from build123d import *

# Parameters (mm, degrees)
F0_W     = 35
F0_H     = 35
F1_DEPTH = 3.5
F2_R     = 2
F3_DEPTH = 7.001
F4_R     = 5
F5_R     = 3.15
F6_DEPTH = 6.3
F7_R     = 2.5
F8_DEPTH = 13.301
F9_SIZE  = 1.4
F10_R    = 0.5


with BuildPart() as f1:
    # F0 (on Top) → F1 (new body, symmetric)
    with BuildSketch(Plane.XY):
        Rectangle(F0_W, F0_H)
    extrude(amount=F1_DEPTH, both=True)

    # F2 (on face) → F3 (cut, through all)
    with BuildSketch(Plane.XY.offset(3.5)):
        with Locations((-12.5, -12.9)):
            Circle(F2_R)
        with Locations((-12.5, 12.5)):
            Circle(F2_R)
        with Locations((12.5, 12.5)):
            Circle(F2_R)
        with Locations((12.5, -12.9)):
            Circle(F2_R)
    extrude(amount=-F3_DEPTH, mode=Mode.SUBTRACT)

    # F4
    f4_edges = [f1.edges().sort_by_distance(p)[0] for p in [
        (-17.5, 17.5, 0),
        (17.5, 17.5, 0),
        (17.5, -17.5, 0),
        (-17.5, -17.5, 0),
    ]]
    fillet(f4_edges, radius=F4_R)

    # F5 (on face) → F6 (join)
    with BuildSketch(Plane.XY.offset(3.5)):
        Circle(F5_R)
    extrude(amount=F6_DEPTH)

    # F7 (on face) → F8 (cut, through all)
    with BuildSketch(Plane.XY.offset(9.8)):
        Circle(F7_R)
    extrude(amount=-F8_DEPTH, mode=Mode.SUBTRACT)

    # F9
    f9_edges = [f1.edges().sort_by_distance(p)[0] for p in [
        (-14.5, -12.9, -3.5),
        (10.5, -12.9, -3.5),
        (10.5, 12.5, -3.5),
        (-14.5, 12.5, -3.5),
    ]]
    chamfer(f9_edges, length=F9_SIZE)

    # F10
    f10_edges = [f1.edges().sort_by_distance(p)[0] for p in [
        (-15.9, -12.9, -3.5),
        (-17.5, 0, -3.5),
    ]]
    fillet(f10_edges, radius=F10_R)


solid = f1.part
Design review of the part built by this model. Coordinates are the model's own, in mm. Coordinates: 2 decimals unless noted, no trailing zeros. Write each loop counter-clockwise with the first axis right and the second up, starting at its lowest first coordinate (ties: lowest second). Pieces come first, ordered by that corner, then holes. Notation, with made-up numbers: (10.25, -32.5) - (43.25, -32.5) arc R25 cw to (43.25, -13.5) - close; hole circle Ø7 at (-16.75, 69). An arc over 180 degrees is marked (long way). One line per item, written item: value.
1) Mouldability with a two-part tool opening along Y and no side actions: class faces 1 (the face through (-16.07, 16, 0.2)), 2 (the face through (-12.76, -10.917, 0.739)), 3 (the face through (0, 4, -3.5)) as +Y half, -Y half, draft (parallel to the pull), parting line (faces both ways), or undercut.
Answer sheet:
face 1: +Y half
face 2: undercut
face 3: draft
2) To check wall thickness, follow probe 1 along Y at (x, z) = (-12.5, 2.3); probe 2 along Z at (x, y) = (14, 4); probe 3 along Y at (x, z) = (-11, -2.25). State the ranges of each line that lie inside material, in increasing order.
Answer sheet:
probe 1: y = -17.5 to -14.9, -10.9 to 10.5, 14.5 to 17.5
probe 2: z = -3.5 to 3.5
probe 3: y = -17.5 to -14.44, -11.36 to 10.96, 14.04 to 17.5
3) Add section D-D (z = 8.25). State the section outline as (x, y) points.
Answer sheet:
outline: circle Ø6.3 at (0, 0); hole circle Ø5 at (0, 0)
4) Add section C-C (y = -0.5). State the section outline as (x, z) points, plus the area to 3 significant figures.
Answer sheet:
outline: (-17.5, -3) arc R0.5 ccw to (-17, -3.5) - (-2.45, -3.5) - (-2.45, 9.8) - (-3.11, 9.8) - (-3.11, 3.5) - (-17.5, 3.5) - close; (2.45, -3.5) - (17, -3.5) arc R0.5 ccw to (17.5, -3) - (17.5, 3.5) - (3.11, 3.5) - (3.11, 9.8) - (2.45, 9.8) - close
area: 219 mm2
5) Insertion check: pin 1 (3 mm diameter, centred on x = -12.5, y = -12.9, fed in from +Z); pin 2 (2 mm diameter, centred on x = 12, y = 0.5, fed in from +Z). Each pin has a flat end and moves straight along its axis. Give the tip position at first contact, or say it passes through.
Answer sheet:
pin 1: passes through
pin 2: stops at z = 3.5
6) Add section A-A (x = 0). State the section outline as (y, z) points, plus the area to 3 significant figures.
Answer sheet:
outline: (-17.5, -3) arc R0.5 ccw to (-17, -3.5) - (-2.5, -3.5) - (-2.5, 9.8) - (-3.15, 9.8) - (-3.15, 3.5) - (-17.5, 3.5) - close; (2.5, -3.5) - (17, -3.5) arc R0.5 ccw to (17.5, -3) - (17.5, 3.5) - (3.15, 3.5) - (3.15, 9.8) - (2.5, 9.8) - close
area: 218 mm2
7) Add section B-B (z = 2). State the section outline as (x, y) points.
Answer sheet:
outline: (-17.5, -12.5) arc R5 ccw to (-12.5, -17.5) - (12.5, -17.5) arc R5 ccw to (17.5, -12.5) - (17.5, 12.5) arc R5 ccw to (12.5, 17.5) - (-12.5, 17.5) arc R5 ccw to (-17.5, 12.5) - close; hole circle Ø4 at (-12.5, -12.9); hole circle Ø4 at (-12.5, 12.5); hole circle Ø5 at (0, 0); hole circle Ø4 at (12.5, -12.9); hole circle Ø4 at (12.5, 12.5)
